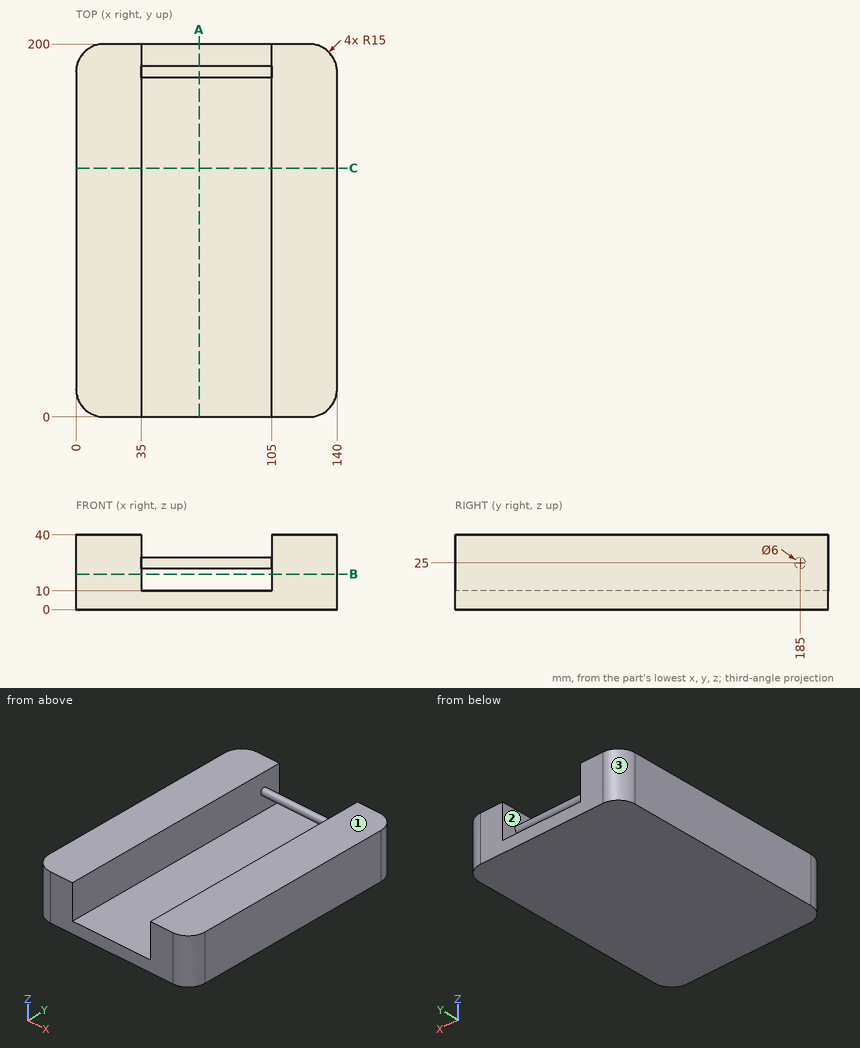
Answer from the drawing. Dimensions are ordinates in mm from the lowest x, y and z of the part. Coordinates: 2 decimals unless noted, no trailing zeros. Loops run counter-clockwise (first coordinate to the right, second up) from the corner with the lowest first, then second, coordinate; pieces in that order, holes last.
Q1. The part is cut by section B-B on z = 19. Write down the section's boundary in (x, y).
Q2. The part is cut by section A-A on x = 66. Write down the section's boundary in (y, z).
Q3. The mould has two halves that part along X. Classify the marked faces 1, 2 and 3: +X half, -X half, draft (parallel to the pull), parting line (faces both ways), or undercut.
Q4. The part is cut by section C-C on y = 133.5. Write down the section's boundary in (x, z).
Q5. Each of these flat-tipped pins is pushed along its axis until it touches: pin 1 Ø6 at (x, y) = (52, 89) entering from +Z; pin 2 Ø4 at (x, z) = (37.5, 15) entering from +Y. Where does it stop, or does it pass through?
Q6. Consider probe 1 along X at (y, z) = (120, 29.5); probe 2 along Z at (x, y) = (53, 171.5); probe 3 along X at (y, z) = (11, 34). Determine where each line is inside the solid, lowest interval first.
Results below:
1. outline: (0, 15) arc R15 ccw to (15, 0) - (35, 0) - (35, 200) - (15, 200) arc R15 ccw to (0, 185) - close; (105, 0) - (125, 0) arc R15 ccw to (140, 15) - (140, 185) arc R15 ccw to (125, 200) - (105, 200) - close
2. outline: (0, 0) - (200, 0) - (200, 10) - (0, 10) - close; circle Ø6 at (185, 25)
3. face 1: draft
3. face 2: undercut
3. face 3: -X half
4. outline: (0, 0) - (140, 0) - (140, 40) - (105, 40) - (105, 10) - (35, 10) - (35, 40) - (0, 40) - close
5. pin 1: stops at z = 10
5. pin 2: passes through
6. probe 1: x = 0 to 35, 105 to 140
6. probe 2: z = 0 to 10
6. probe 3: x = 0.54 to 35, 105 to 139.46
